For this review, take the finished solid that the model builds, in its own axes (mm). Face numbers are marked on the shaded views. A direction names the side the tool comes from. Round coordinates to 2 decimals unless told otherwise and drop trailing zeros. Order: outer loops, then holes, each group sorted by start corner. A loop starts at its lowest first (then second) coordinate and runs counter-clockwise, first axis right, second up. Notation, with made-up numbers: M 23.5,84 L 63.5,84 A19 cw 63.5,108 Z; hole C 56,54 d1. An arc over 180 degrees is marked long. Answer as a JSON object with one key per item and string values.
from build123d import *

# Parameters (mm, degrees)
SKETCH_2_W          = 1
SKETCH_2_H          = 5.907580982
CUT_EXTRUDE_1_DEPTH = 1.2
SKETCH_3_R          = 1.5
EXTRUDE_2_DEPTH     = 5


with BuildPart() as part:
    # Эскиз1 → Повернуть1 (revolve)
    with BuildSketch(Plane.XY):
        with BuildLine():
            Line((0, 0), (2.65, 0))
            ThreePointArc((2.65, 0), (1.630375724, 1.375918772), (0, 1.9))
            Line((0, 1.9), (0, 0))
        make_face()
    revolve(axis=Axis((0, 0, 0), (0, 1, 0)))

    # Эскиз2 → Вытянуть1 (cut)
    with BuildSketch(Plane(origin=(0, 2, 0), x_dir=(1, 0, 0), z_dir=(0, 1, 0))):
        Rectangle(SKETCH_2_W, SKETCH_2_H)
    extrude(amount=-CUT_EXTRUDE_1_DEPTH, mode=Mode.SUBTRACT)

    # Эскиз3 → Вытянуть2 (add)
    with BuildSketch(Plane.XZ):
        with Locations(Location((0, 0, 0), (0, 0, 270))):
            Circle(SKETCH_3_R)
    extrude(amount=EXTRUDE_2_DEPTH)


solid = part.part
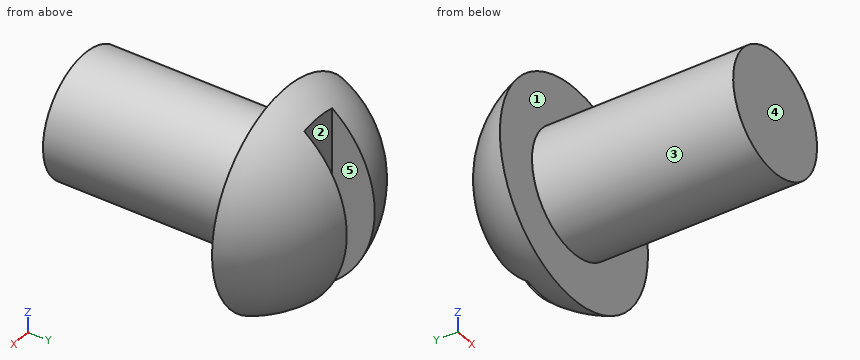
1) Mouldability with a two-part tool opening along X and no side actions: class the marked faces 3, 4 and 5 as +X half, -X half, draft (parallel to the pull), parting line (faces both ways), or undercut.
Geometry check:
{"face 3": "parting line", "face 4": "draft", "face 5": "undercut"}
2) Insertion check: P1, Ø1, axis at x = 1, y = -4, coming from the +Z side; P2, Ø1, axis at y = -2, z = -1.5, coming from the +X side; P3, Ø0.5, axis at y = 1.5, z = -1, coming from the -X side. Each pin has a flat end and moves straight along its axis. Give the tip position at first contact, or say it passes through.
Geometry check:
{"P1": "stops at z = 1.41", "P2": "stops at x = 1.12", "P3": "stops at x = -1.52"}
3) Add section D-D on y = 1. State the section outline as (x, z) points, and give its area (3 significant figures).
Geometry check:
{"outline": "M -0.5,-1.99 L -0.5,1.99 A2.06 ccw Z; M 0.5,-1.99 A2.06 ccw 0.5,1.99 Z", "area": "9.21 mm²"}
4) Add section A-A on x = 0. State the section outline as (y, z) points.
Geometry check:
{"outline": "M -5,-1.5 L 0,-1.5 L 0,-2.65 A2.8 ccw 0.8,-2.22 L 0.8,2.22 A2.8 ccw 0,2.65 L 0,1.5 L -5,1.5 Z"}
5) Add section B-B on z = 0. State the section outline as (x, y) points.
Geometry check:
{"outline": "M -2.65,0 L -1.5,0 L -1.5,-5 L 1.5,-5 L 1.5,0 L 2.65,0 A2.8 ccw 0.5,1.85 L 0.5,0.8 L -0.5,0.8 L -0.5,1.85 A2.8 ccw Z"}
6) For L1, parallel to X at y = 1, z = 0.25; L2, parallel to Y at x = 0.2, z = 0.8; L3, parallel to Y at x = 2.35, z = -0.05, list the stretches that pass through material, from the lowest coordinate up.
Geometry check:
{"L1": "x = -2.04 to -0.5, 0.5 to 2.04", "L2": "y = -5 to 0.8", "L3": "y = 0 to 0.62"}
7) Machinability: for the marked faces 1 and 2, which of the approach directions +Z, -Z, +X, -X, +Y, -Y give a long, thin tool a straight path to every point of the face, cutting with its end or side? Answer none if there is none.
Geometry check:
{"face 1": "-Y", "face 2": "+Z, -Z, +Y"}
8) Add section C-C on y = -4. State the section outline as (x, z) points, and give its area (3 significant figures).
Geometry check:
{"outline": "C 0,0 d3", "area": "7.07 mm²"}
